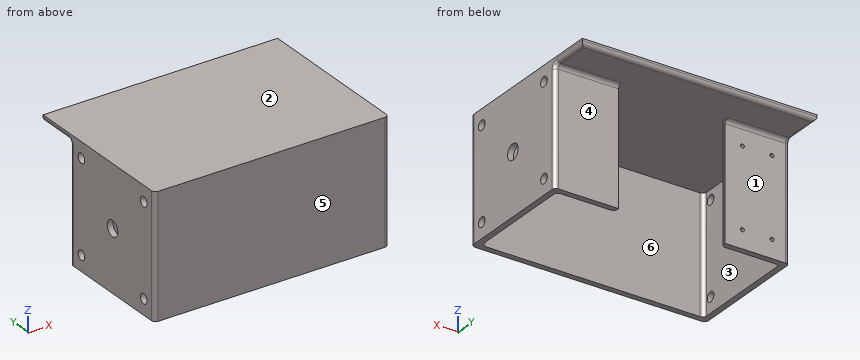
Autodesk Inventor part; units mm, degrees
ref_plane "YZ Plane" through (0, 0, 0) normal (1, 0, 0) x (0, 1, 0)
ref_plane "XZ Plane" through (0, 0, 0) normal (0, 1, 0) x (-1, 0, 0)
ref_plane "XY Plane" through (0, 0, 0) normal (0, 0, 1) x (1, 0, 0)
sketch "Boceto1" plane through (0, 0, 0) normal (0, 0, 1) x (1, 0, 0)
  line L0 (105, 0) -> (105, 24.5)
  line L1 (0, 24.5) -> (0, 0)
  line L2 (105, 24.5) -> (0, 24.5)
  line L3 (113, 129.5) -> (-8, 129.5)
  line L4 (-8, 129.5) -> (-8, -80.5)
  line L5 (-8, -80.5) -> (113, -80.5)
  line L6 (113, -80.5) -> (113, 129.5)
  line L7 (113, 129.5) -> (-8, -80.5) construction
  line L8 (-8, 129.5) -> (113, -80.5) construction
  point P0 (52.5, 24.5)
  dimension "d0" = 121
  dimension "d1" = 210
extrude "Extrusión1" add sketch "Boceto1" along normal blind 3
sketch "Boceto2" plane through (0, 0, 0) normal (0, 0, -1) x (-1, 0, 0)
  line L0 (0, 53) -> (5, 53)
  line L1 (0, -4) -> (5, -4)
  line L2 (5, 53) -> (8, 53)
  line L3 (8, 129.5) -> (8, -80.5)
  line L4 (5, -4) -> (8, -4)
  line L5 (8, -4) -> (8, 53)
  line L6 (8, 53) -> (5, 53)
  line L7 (5, 53) -> (5, -4)
  point P0 (0, 0)
ref_plane "Plano de trabajo1" through (52.5, -80.5, 0) normal (-1, 0, 0) x (0, 0, 1)
extrude "Extrusión2" add sketch "Boceto2" along normal blind 60
sketch "Boceto3" plane through (-8, -80.5, 3) normal (-1, 0, 0) x (0, 0, 1)
  circle A0 centre (-54.9977, 81.5) radius 3
  circle A1 centre (-54.9977, 128.5) radius 3
  circle A2 centre (-7.9977, 128.5) radius 3
  circle A3 centre (-7.9977, 81.5) radius 3
  point P0 (-3, 80.5)
hole "Agujero1" at (-8, 1, -51.9977) at (-8, 48, -51.9977) at (-8, 48, -4.9977) at (-8, 1, -4.9977) direction (1, 0, 0) diameter 5 end up to surface
sketch "Boceto4" plane through (-8, -80.5, 3) normal (-1, 0, 0) x (0, 0, 1)
  circle A0 centre (-31.4977, 105) radius 4
  circle A1 centre (-31.4977, 105) radius 4
  point P0 (-3, 80.5)
  dimension "d13" = 8
hole "Agujero2" at (-8, 24.5, -28.4977) direction (1, 0, 0) diameter 8 end up to surface
sketch "Boceto5" plane through (-8, 53, 0) normal (0, 1, 0) x (1, 0, 0)
  line L0 (3, 0) -> (33, 0)
  line L1 (33, 0) -> (33, 60)
  line L2 (33, 60) -> (3, 60)
  line L3 (3, 60) -> (0, 60)
  line L4 (0, 60) -> (0, 0)
  line L5 (0, 0) -> (3, 0)
  line L6 (33, 60) -> (33, 0)
  line L7 (33, 60) -> (0, 60)
  line L8 (0, 60) -> (0, 0)
  line L9 (0, 0) -> (33, 0)
  line L10 (33, 0) -> (33, 60)
  point P0 (8, 0)
  dimension "d21" = 30
  dimension "d22" = 60
extrude "Extrusión3" add sketch "Boceto5" along normal blind 3
sketch "Boceto6" plane through (-8, 56, 0) normal (0, 1, 0) x (1, 0, 0)
  circle A0 centre (8.88, 50.6734) radius 0.889
  circle A1 centre (24.12, 50.6734) radius 0.889
  circle A2 centre (24.12, 10.0334) radius 0.889
  circle A3 centre (8.88, 10.0334) radius 0.889
  point P0 (8, 0)
hole "Agujero3" at (16.12, 56, -50.6734) at (0.88, 56, -50.6734) at (16.12, 56, -10.0334) at (0.88, 56, -10.0334) direction (0, -1, 0) diameter 2 end up to surface
mirror "Simetría1" about plane through (52.5, -80.5, 0) normal (-1, 0, 0) of "Extrusión3", "Agujero2", "Agujero1", "Extrusión2"
fillet "Empalme1" radius 2 2 edges at (96.5, 56, 0) (8.5, 56, 0)
sketch "Boceto7" plane through (0, 0, 0) normal (0, 0, -1) x (-1, 0, 0)
  line L0 (8, -4) -> (8, -7)
  line L1 (8, -4) -> (8, -80.5)
  line L2 (8, -7) -> (-113, -7)
  line L3 (-113, -80.5) -> (-113, 129.5)
  line L4 (-113, -80.5) -> (-113, -7)
  line L5 (-113, -80.5) -> (-113, -4)
  line L6 (-113, -80.5) -> (8, -80.5)
  line L7 (8, -80.5) -> (8, -7)
  point P0 (0, 0)
  dimension "d33" = 3
extrude "Extrusión4" cut sketch "Boceto7" against normal blind 3
sketch "Boceto8" plane through (0, 0, 0) normal (0, 0, -1) x (-1, 0, 0)
  line L0 (-113, -4) -> (-113, -7)
  line L1 (-113, -7) -> (8, -7)
  line L2 (8, -7) -> (8, -4)
  line L3 (8, -4) -> (-113, -4)
  point P0 (0, 0)
  dimension "d36" = 3
  dimension "d37" = 121
  dimension "d38" = 3
extrude "Extrusión5" add sketch "Boceto8" along normal blind 60
sketch "Boceto9" plane through (0, 0, -60) normal (0, 0, -1) x (-1, 0, 0)
  point P0 (0, 0)
sketch "Boceto10" plane through (0, 0, 0) normal (0, 0, -1) x (-1, 0, 0)
  line L0 (-46.8669, 72) -> (-100.1331, 72)
  line L1 (-46.8669, 77) -> (-100.1331, 77)
  line L2 (-100.1331, 77) -> (-113, 77)
  line L3 (-113, 58) -> (-113, 129.5)
  line L4 (-46.8669, 77) -> (6.9064, 77)
  line L5 (6.9064, 77) -> (8, 77)
  line L6 (8, 129.5) -> (8, 58)
  line L7 (-113, 77) -> (8.9757, 77)
  line L8 (8.9757, 77) -> (8.9757, 129.5)
  line L9 (8.9757, 129.5) -> (-113, 129.5)
  line L10 (-113, 129.5) -> (-113, 77)
  point P0 (0, 0)
  dimension "d41" = 5
extrude "Extrusión6" cut sketch "Boceto10" against normal blind 10
fillet "Empalme2" radius 2 11 edges at (-5, 53, -30) (-8, 56.5858, -0.5858) (-8, 67.5, 0) (-8, 56, -31) (-5, -4, -30) (110, -4, -30) (110, 53, -30) (113, 56.5858, -0.5858) (113, 67.5, 0) (113, 56, -31) (52.5, 77, 0)
fillet "Empalme3" radius 2 2 edges at (80, 53, -30) (25, 53, -30)
fillet "Empalme4" radius 2 2 edges at (113, -7, -28.5) (-8, -7, -28.5)
properties part number "base"
Read the model definition and answer for the solid it produces. Units are mm, in the model's axes. Face numbers are marked on the shaded views. A direction names the side the tool comes from. Round coordinates to 2 decimals unless told otherwise and drop trailing zeros. Loops run counter-clockwise (first coordinate to the right, second up) from the corner with the lowest first, then second, coordinate; pieces in that order, holes last.
Q1. Section A-A on y = 48 is taken. Write down the section's boundary in (x, z), and give its area (3 significant figures).
Q2. Which of the six approach directions +Z, -Z, +X, -X, +Y, -Y give full straight-line access (tool end or side, diameter ignored) to the marked faces 1, 2 and 3?
Q3. Consider probe 1 along Z at (x, y) = (111, 1); probe 2 along Y at (x, z) = (11, -15.5); probe 3 along X at (y, z) = (8, -18). Determine where each line is inside the solid, lowest interval first.
Q4. Each of these flat-tipped pins is pushed along its axis until it touches: pin 1 (12 mm diameter, centred on x = 65.5, y = 17.5, fed in from -Z); pin 2 (1.8 mm diameter, centred on x = 16.12, z = -50.67, fed in from +Y); pin 3 (6.5 mm diameter, centred on y = 48, z = -52, fed in from -X); pin 4 (6 mm diameter, centred on x = 8, z = -10, fed in from +Y). Where does it stop, or does it pass through?
Q5. Determine the mould class of the marked faces 4, 5 and 6 for opening direction Y: released by +Y, released by -Y, zero draft, split by the parting line, or undercut.
Q6. Section D-D on z = -39.5 is taken. Write down the section's boundary in (x, y), and give its area (3 significant figures).
Q7. Section C-C on x = 31 is taken. Write down the section's boundary in (y, z), and give its area (3 significant figures).
Q8. Section B-B on y = 24.5 is taken. Write down the section's boundary in (x, z), and give its area (3 significant figures).
Output:
1. outline: (-8, -60) - (-5, -60) - (-5, -54.5) - (-8, -54.5) - close; (-8, -49.5) - (-5, -49.5) - (-5, -7.5) - (-8, -7.5) - close; (-8, -2.5) - (-5, -2.5) - (-5, 0) - (110, 0) - (110, -2.5) - (113, -2.5) - (113, 3) - (-8, 3) - close; (110, -60) - (113, -60) - (113, -54.5) - (110, -54.5) - close; (110, -49.5) - (113, -49.5) - (113, -7.5) - (110, -7.5) - close
1. area: 663 mm2
2. face 1: -Z, +X, -X, +Y
2. face 2: +Z, +X, -X, +Y, -Y
2. face 3: -Z
3. probe 1: z = -60 to -54.5, -49.5 to -7.5, -2.5 to 3
3. probe 2: y = -7 to -4, 53 to 56
3. probe 3: x = -8 to -5, 110 to 113
4. pin 1: stops at z = 0
4. pin 2: stops at y = -4
4. pin 3: stops at x = -8
4. pin 4: stops at y = 56
5. face 4: released by +Y
5. face 5: released by -Y
5. face 6: undercut
6. outline: (-8, -5) arc R2 ccw to (-6, -7) - (111, -7) arc R2 ccw to (113, -5) - (113, 54) arc R2 ccw to (111, 56) - (80, 56) - (80, 55) arc R2 ccw to (82, 53) - (108, 53) arc R2 cw to (110, 51) - (110, -2) arc R2 cw to (108, -4) - (-3, -4) arc R2 cw to (-5, -2) - (-5, 51) arc R2 cw to (-3, 53) - (23, 53) arc R2 ccw to (25, 55) - (25, 56) - (-6, 56) arc R2 ccw to (-8, 54) - close
6. area: 901 mm2
7. outline: (-7, -60) - (-4, -60) - (-4, 0) - (75, 0) arc R2 ccw to (77, 2) - (77, 3) - (-7, 3) - close
7. area: 431 mm2
8. outline: (-8, -60) - (-5, -60) - (-5, -32.5) - (-8, -32.5) - close; (-8, -24.5) - (-5, -24.5) - (-5, 0) - (110, 0) - (110, -24.5) - (113, -24.5) - (113, 3) - (-8, 3) - close; (110, -60) - (113, -60) - (113, -32.5) - (110, -32.5) - close
8. area: 675 mm2
